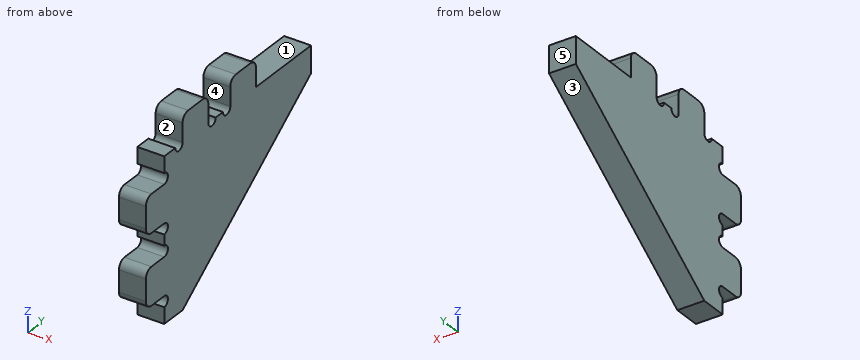
```python
from build123d import *

# Parameters (mm, degrees)
EXTRUDE_1_DEPTH     = 5
SKETCH_2_W          = 7
SKETCH_2_H          = 5
SKETCH_2_W_2        = 5
SKETCH_2_H_2        = 7
EXTRUDE_2_DEPTH     = 5
SKETCH_3_R          = 1
CUT_EXTRUDE_1_DEPTH = 5
FILLET_1_R          = 1.5


with BuildPart() as part:
    # 스케치1 → 보스-돌출1 (new body)
    with BuildSketch(Plane(origin=(0, 0, 0), x_dir=(0, 0, -1), z_dir=(1, 0, 0))):
        Polygon((0, 0), (0, 40), (5, 40), (30, 5), (30, 0), align=None)
    extrude(amount=EXTRUDE_1_DEPTH)

    # 스케치2 → 보스-돌출2 (add)
    with BuildSketch(Plane(origin=(5, 0, 0), x_dir=(0, 0, -1), z_dir=(1, 0, 0))):
        with Locations((8.5, -2.5)):
            Rectangle(SKETCH_2_W, SKETCH_2_H)
        with Locations((21.5, -2.5)):
            Rectangle(SKETCH_2_W, SKETCH_2_H)
        with Locations((-2.5, 21.5)):
            Rectangle(SKETCH_2_W_2, SKETCH_2_H_2)
        with Locations((-2.5, 8.5)):
            Rectangle(SKETCH_2_W_2, SKETCH_2_H_2)
    extrude(amount=-EXTRUDE_2_DEPTH)

    # 스케치3 → 컷-돌출1 (cut)
    with BuildSketch(Plane(origin=(5, 0, 0), x_dir=(0, 0, -1), z_dir=(1, 0, 0))):
        with Locations((4, 0)):
            Circle(SKETCH_3_R)
        with Locations((13, 0)):
            Circle(SKETCH_3_R)
        with Locations((17, 0)):
            Circle(SKETCH_3_R)
        with Locations((26, 0)):
            Circle(SKETCH_3_R)
        with Locations((0, 4)):
            Circle(SKETCH_3_R)
        with Locations((0, 13)):
            Circle(SKETCH_3_R)
        with Locations((0, 17)):
            Circle(SKETCH_3_R)
    extrude(amount=-CUT_EXTRUDE_1_DEPTH, mode=Mode.SUBTRACT)

    # 필렛1
    fillet_1_edges = [part.edges().sort_by_distance(p)[0] for p in [
        (2.5, -5, -25),
        (2.5, -5, -12),
        (2.5, -5, -18),
        (2.5, 25, 5),
        (2.5, 18, 5),
        (2.5, -5, -5),
        (2.5, 5, 5),
        (2.5, 12, 5),
    ]]
    fillet(fillet_1_edges, radius=FILLET_1_R)


solid = part.part
```
For this review, take the finished solid that the model builds, in its own axes (mm). Face numbers are marked on the shaded views. A direction names the side the tool comes from. Coordinates: 2 decimals unless noted, no trailing zeros. Loops run counter-clockwise (first coordinate to the right, second up) from the corner with the lowest first, then second, coordinate; pieces in that order, holes last.
1. Add section A-A, the plane z = 1. Give the boundary of the cut face in (x, y), then the cut area to 3 significant figures.
2. Add section C-C, the plane y = 13. Give the boundary of the cut face in (x, z), then the cut area to 3 significant figures.
3. Add section B-B, the plane z = -26. Give the boundary of the cut face in (x, y).
4. Insertion check: P1, Ø1, axis at x = 2.5, y = -1, coming from the -Z side; P2, Ø2, axis at x = 2, z = -12.5, coming from the -Y side; P3, Ø3, axis at x = 3.5, z = 2, coming from the +Y side; P4, Ø3, axis at x = 1.5, z = 1, coming from the +Y side. Each pin has a flat end and moves straight along its axis. Give the tip position at first contact, or say it passes through.
5. For the marked faces 1, 2, 3, 4 and 5, list the 3-axis set-ups (+Z, -Z, +X, -X, +Y, -Y) from which the entire face can be reached by the end or side of a thin tool; tool diameter is ignored.
6. For line 1 (Y direction, x = 3.45, z = 2); line 2 (Z direction, x = 1.4, y = -2.5); line 3 (Y direction, x = 0.6, z = -2), list the stretches that pass through material, from the lowest coordinate up.
Result:
1. outline: (0, 5) - (5, 5) - (5, 12) - (0, 12) - close; (0, 18) - (5, 18) - (5, 25) - (0, 25) - close
1. area: 70.0 mm2
2. outline: (0, -24.29) - (5, -24.29) - (5, -1) - (0, -1) - close
2. area: 116 mm2
3. outline: (0, 1) - (5, 1) - (5, 10.6) - (0, 10.6) - close
4. P1: stops at z = -25
4. P2: stops at y = -4.62
4. P3: stops at y = 25
4. P4: stops at y = 40
5. face 1: +Z, +X, -X, +Y
5. face 2: +Z, +X, -X, -Y
5. face 3: -Z, +X, -X, +Y
5. face 4: +Z, +X, -X
5. face 5: +Z, -Z, +X, -X, +Y
6. line 1: y = 5 to 12, 18 to 25
6. line 2: z = -25 to -18, -12 to -5
6. line 3: y = 0 to 40
